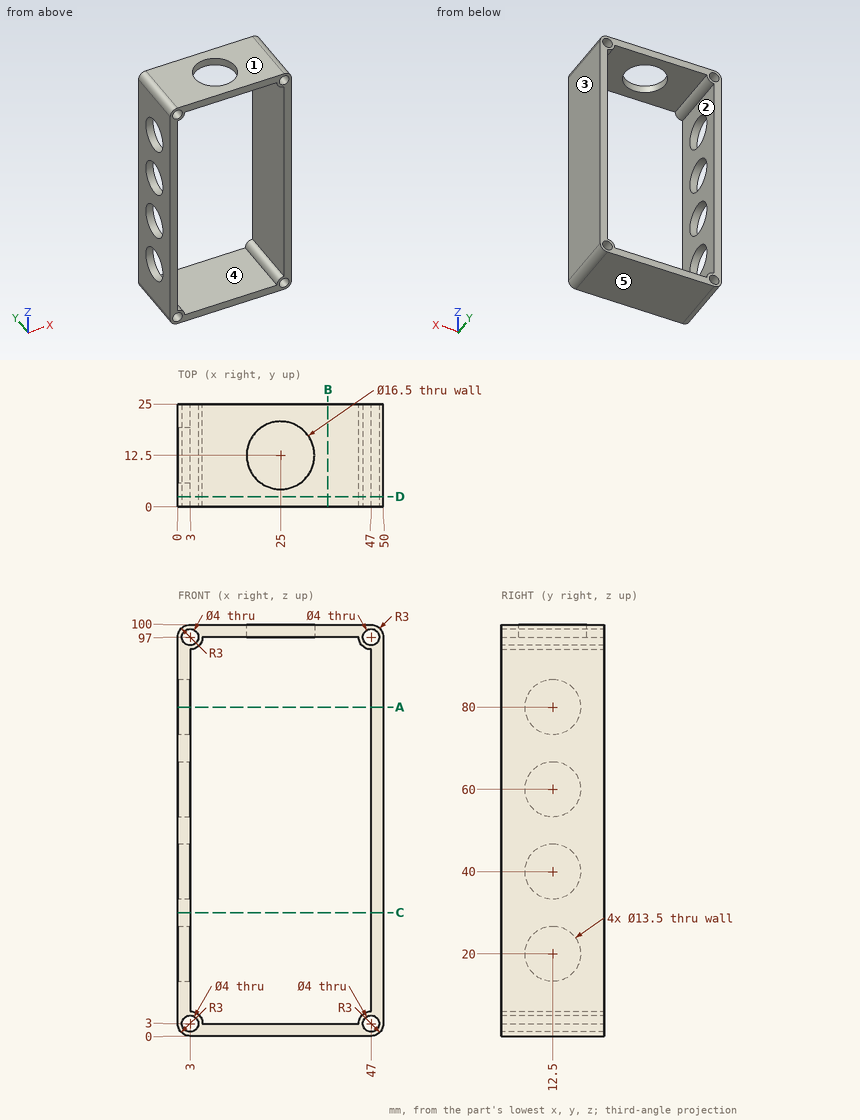
Geometry: see drawing. Coordinates: mm, zero at the bounding-box minimum. A direction names the side the tool comes from. Round coordinates to 2 decimals unless told otherwise and drop trailing zeros. Write each loop counter-clockwise with the first axis right and the second up, starting at its lowest first coordinate (ties: lowest second). Pieces come first, ordered by that corner, then holes.
1) Draft query along X for the marked faces 1, 2 and 3. Return one class per face: pulls with the +X half, pulls with the -X half, needs draft (parallel to the pull), parting line crosses it, or undercut.
2) Cut plane B-B (x = 36.5). Return the cut outline in (y, z), then the cut area to 3 significant figures.
3) Cut plane C-C (z = 30). Return the cut outline in (x, y).
4) Contact query for a flat-ended pin moving along its axis: P1, Ø8, axis at y = 12.5, z = 20, coming from the -X side. Output: stop coordinate, or through.
5) Cut plane A-A (z = 80). Return the cut outline in (x, y).
6) Reachability of the marked faces 4 and 5 from +Z, -Z, +X, -X, +Y, -Y: full face, straight path, thin tool, end or side. Return the list, or none.
7) Cut plane D-D (y = 2.5). Return the cut outline in (x, z), then the cut area to 3 significant figures.
8) Ray query, L1, parallel to Y at x = 1.85, z = 40; L2, parallel to X at y = 17.25, z = 47; L3, parallel to Z at x = 38, y = 15.75. Return the intervals inside material, ascending.
Geometry says:
1. face 1: needs draft
1. face 2: undercut
1. face 3: pulls with the +X half
2. outline: (0, 0) - (25, 0) - (25, 3) - (0, 3) - close; (0, 97) - (25, 97) - (25, 100) - (0, 100) - close
2. area: 150 mm2
3. outline: (0, 0) - (3, 0) - (3, 25) - (0, 25) - close; (47, 0) - (50, 0) - (50, 25) - (47, 25) - close
4. P1: stops at x = 47
5. outline: (0, 0) - (3, 0) - (3, 5.75) - (0, 5.75) - close; (0, 19.25) - (3, 19.25) - (3, 25) - (0, 25) - close; (47, 0) - (50, 0) - (50, 25) - (47, 25) - close
6. face 4: +Y, -Y
6. face 5: -Z, +X, -X, +Y, -Y
7. outline: (0, 3) arc R3 ccw to (3, 0) - (47, 0) arc R3 ccw to (50, 3) - (50, 97) arc R3 ccw to (47, 100) - (3, 100) arc R3 ccw to (0, 97) - close; hole circle Ø4 at (3, 3); hole circle Ø4 at (3, 97); hole (3, 6) arc R3 cw to (6, 3) - (44, 3) arc R3 cw to (47, 6) - (47, 94) arc R3 cw to (44, 97) - (6, 97) arc R3 cw to (3, 94) - close; hole circle Ø4 at (47, 3); hole circle Ø4 at (47, 97)
7. area: 834 mm2
8. L1: y = 0 to 5.75, 19.25 to 25
8. L2: x = 0 to 3, 47 to 50
8. L3: z = 0 to 3, 97 to 100
